Study the drawing (mm; zero at the part's minimum x, y, z) and answer. Coordinates: 2 decimals unless noted, no trailing zeros. Order: outer loops, then holes, each group sorted by start corner. A loop starts at its lowest first (then second) coordinate and runs counter-clockwise, first axis right, second up.
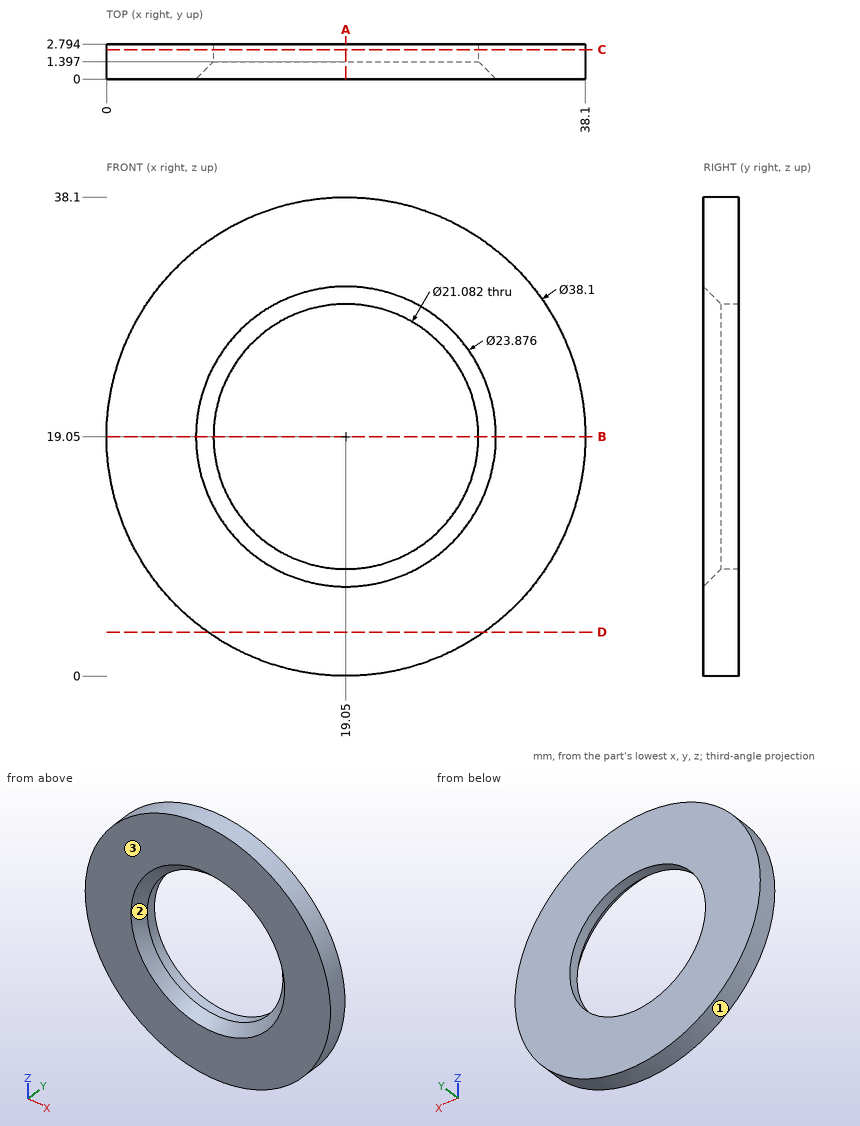
1) A cutting plane is placed at A-A, the plane x = 19.05. Determine the outline of the cut face in (y, z).
A:
outline: (0, 0) - (2.79, 0) - (2.79, 8.51) - (1.4, 8.51) - (0, 7.11) - close; (0, 30.99) - (1.4, 29.59) - (2.79, 29.59) - (2.79, 38.1) - (0, 38.1) - close
2) Determine the mould class of the marked faces 1, 2 and 3 for opening direction X: pulls with the +X half, pulls with the -X half, needs draft (parallel to the pull), parting line crosses it, or undercut.
A:
face 1: parting line crosses it
face 2: undercut
face 3: needs draft
3) A cutting plane is placed at B-B, the plane z = 19.05. Determine the outline of the cut face in (x, y).
A:
outline: (0, 0) - (7.11, 0) - (8.51, 1.4) - (8.51, 2.79) - (0, 2.79) - close; (29.59, 1.4) - (30.99, 0) - (38.1, 0) - (38.1, 2.79) - (29.59, 2.79) - close
4) Straight lines are drawn through the part: line 1 (Z direction, x = 19.05, y = 2.35); line 2 (Z direction, x = 17.5, y = 1.35); line 3 (X direction, y = 0.4, z = 25). For each, find the intervals that lie inside material, in ascending order.
A:
line 1: z = 0 to 8.51, 29.59 to 38.1
line 2: z = 0.06 to 8.58, 29.52 to 38.04
line 3: x = 0.95 to 9.16, 28.94 to 37.15
5) Flat-ended cylindrical pins translate along their axes: pin 1 Ø1 at (y, z) = (0.5, 12) entering from +X; pin 2 Ø1.5 at (y, z) = (2, 8) entering from +X; pin 3 Ø1.5 at (x, y) = (11, 0.5) entering from -Z. Find the tip coordinate at first contact, or state that the pin passes through.
A:
pin 1: stops at x = 36.94
pin 2: stops at x = 35.08
pin 3: stops at z = 1.45
6) A cutting plane is placed at C-C, the plane y = 2.35. Determine the outline of the cut face in (x, z), and give its area (3 significant figures).
A:
outline: circle Ø38.1 at (19.05, 19.05); hole circle Ø21.08 at (19.05, 19.05)
area: 791 mm2
7) A cutting plane is placed at D-D, the plane z = 3.5. Determine the outline of the cut face in (x, y), and give its area (3 significant figures).
A:
outline: (8.05, 0) - (30.05, 0) - (30.05, 2.79) - (8.05, 2.79) - close
area: 61.5 mm2
